Autodesk Inventor part; units mm, degrees
ref_plane "YZ Plane" through (0, 0, 0) normal (1, 0, 0) x (0, 1, 0)
ref_plane "XZ Plane" through (0, 0, 0) normal (0, 1, 0) x (-1, 0, 0)
sketch "Sketch3" plane through (0, 0, 0) normal (0, 0, 1) x (1, 0, 0)
  line L0 (0, -9.525) -> (9.525, -9.525)
  line L1 (9.525, -9.525) -> (9.525, 0)
  line L2 (0, 0) -> (0, -9.525) construction
  line L3 (0, 0) -> (9.525, 0) construction
  line L4 (0, -9.525) -> (-9.525, -9.525)
  line L5 (-9.525, -9.525) -> (-9.525, 0)
  line L6 (9.525, 0) -> (73.025, 0)
  line L7 (-187.325, 0) -> (-187.325, 19.05)
  line L8 (-187.325, 0) -> (-9.525, 0)
  line L9 (73.025, 0) -> (73.025, 19.05)
  line L10 (73.025, 19.05) -> (-187.325, 19.05)
  dimension "d0" = 9.525
  dimension "d1" = 9.525
  dimension "d6" = 63.5
  dimension "d8" = 19.05
  dimension "d9" = 177.8
extrude "Extrusion1" add sketch "Sketch3" along normal mid plane 355.6
sketch "Sketch4" plane through (0, 0, 177.8) normal (0, 0, 1) x (1, 0, 0)
  line L0 (-187.325, 19.05) -> (73.025, 19.05) construction
  line L1 (0, 19.05) -> (0, -9.525) construction
  line L2 (9.525, -9.525) -> (-9.525, -9.525) construction
  line L3 (0, -9.525) -> (-22.225, -9.525)
  line L4 (-22.225, -9.525) -> (-22.225, 19.05)
  line L5 (-22.225, 19.05) -> (0, 19.05)
  line L6 (187.325, 19.05) -> (-73.025, 19.05) construction
  line L7 (0, -9.525) -> (22.225, -9.525)
  line L8 (22.225, -9.525) -> (22.225, 19.05)
  line L9 (0, 19.05) -> (22.225, 19.05)
  point P0 (0, 0)
  dimension "d12" = 22.225
extrude "Extrusion2" add sketch "Sketch4" along normal blind 12.7
mirror "Mirror1" about plane through (0, 0, 0) normal (0, 0, 1) of "Extrusion2"
sketch "Sketch6" plane through (-187.325, 0, -177.8) normal (0, -1, 0) x (1, 0, 0)
  line L0 (82.55, 165.1) -> (88.9, 165.1)
  line L1 (88.9, 165.1) -> (88.9, 190.5)
  line L2 (88.9, 190.5) -> (82.55, 190.5)
  line L3 (82.55, 190.5) -> (82.55, 165.1)
  line L4 (82.55, 165.1) -> (88.9, 190.5) construction
  line L5 (88.9, 165.1) -> (82.55, 190.5) construction
  line L6 (177.8, 0) -> (177.8, 355.6)
  point P0 (187.325, 177.8)
  point P1 (85.725, 177.8)
  dimension "d16" = 12.7
  dimension "d18" = 6.35
  dimension "d19" = 88.9
extrude "Extrusion3" cut sketch "Sketch6" against normal through all
sketch "Sketch7" plane through (0, 0, 177.8) normal (0, 0, 1) x (1, 0, 0)
  line L0 (-187.325, 19.05) -> (-22.225, 19.05)
  line L1 (-161.925, 19.05) -> (-117.475, 19.05)
  line L2 (-117.475, 19.05) -> (-117.475, -3.81)
  line L3 (-117.475, -3.81) -> (-161.925, -3.81)
  line L4 (-161.925, -3.81) -> (-161.925, 19.05)
  line L5 (-187.325, 19.05) -> (-187.325, 0)
  point P0 (0, 0)
  dimension "d22" = 44.45
  dimension "d23" = 22.86
  dimension "d24" = 25.4
extrude "Extrusion4" add sketch "Sketch7" along normal blind 12.7
mirror "Mirror2" about plane through (0, 0, 0) normal (0, 0, 1) of "Extrusion4"
sketch "Sketch9" plane through (73.025, 0, 177.8) normal (1, 0, 0) x (0, 0, -1)
  line L0 (355.6, 19.05) -> (0, 19.05)
  line L1 (50.8, 19.05) -> (63.5, 19.05)
  line L2 (63.5, 19.05) -> (63.5, 12.7)
  line L3 (63.5, 12.7) -> (50.8, 12.7)
  line L4 (50.8, 12.7) -> (50.8, 19.05)
  line L5 (0, 0) -> (0, 19.05)
  point P0 (177.8, 0)
  dimension "d28" = 12.7
  dimension "d29" = 6.35
  dimension "d30" = 50.8
extrude "Extrusion5" cut sketch "Sketch9" against normal through all
mirror "Mirror3" about plane through (0, 0, 0) normal (0, 0, 1) of "Extrusion5"
sketch "Sketch12" plane through (73.025, 0, 177.8) normal (1, 0, 0) x (0, 0, -1)
  line L0 (355.6, 0) -> (0, 0) construction
  line L1 (88.9, 0) -> (88.9, 16.5009) construction
  line L2 (0, 0) -> (0, 19.05)
  line L3 (50.8, 19.05) -> (0, 19.05)
  line L4 (84.1375, 19.05) -> (84.1375, 12.7)
  line L5 (84.1375, 12.7) -> (80.1624, 12.7)
  line L6 (80.1624, 12.7) -> (80.1624, 6.35)
  line L7 (80.1624, 6.35) -> (88.9, 6.35)
  line L8 (93.6625, 19.05) -> (93.6625, 12.7)
  line L9 (93.6625, 12.7) -> (97.6376, 12.7)
  line L10 (97.6376, 12.7) -> (97.6376, 6.35)
  line L11 (97.6376, 6.35) -> (88.9, 6.35)
  line L12 (84.1375, 19.05) -> (93.6625, 19.05)
  point P0 (177.8, 0)
  dimension "d46" = 88.9
  dimension "d47" = 4.7625
  dimension "d48" = 6.35
  dimension "d49" = 6.35
  dimension "d50" = 8.7376
extrude "Extrusion8" cut sketch "Sketch12" against normal through all
mirror "Mirror4" about plane through (0, 0, 0) normal (0, 0, 1) of "Extrusion8"
split "Split2" plane through (0, 0, 0) removes the side toward (0, 0, -1)
ref_plane "Work Plane1" through (-60.325, 0, 177.8) normal (1, 0, 0) x (0, 0, -1)
properties part number "BandSawJigBottomSpiltA" material "LCP Plastic"
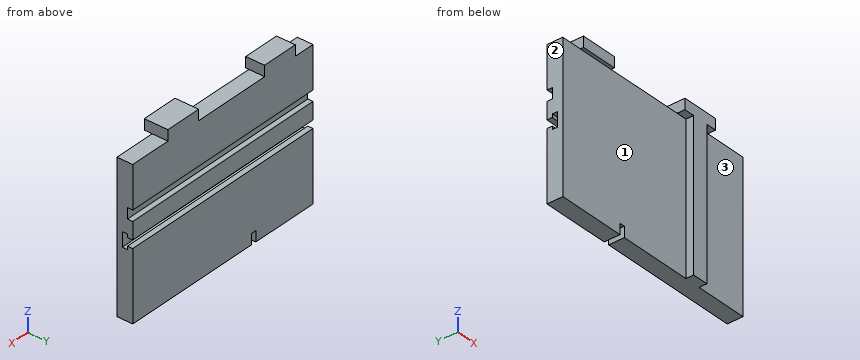
Verification items for the finished model (mm, model axes). Face numbers are marked on the shaded views. A direction names the side the tool comes from. Coordinates: 2 decimals unless noted, no trailing zeros. Order: outer loops, then holes, each group sorted by start corner. A loop starts at its lowest first (then second) coordinate and runs counter-clockwise, first axis right, second up. Notation, with made-up numbers: (80, -17.75) -> (113, -17.75) arc R23 ccw to (113, 8.25) -> close; hole circle Ø4 at (82, 2). An arc over 180 degrees is marked (long way). Use CSV: the item, a comma, the result in double quotes. Start each with the question number.
Q1. Section check D-D, the plane z = 43. Record the cut outline in (x, y) (3 decimals).
Q2. Section check C-C, the plane y = 2.75. Record the cut outline in (x, z) (3 decimals), and give its area (3 significant figures).
Q3. Depth check by flat-ended pin: P1, Ø5, axis at x = 2.5, y = -5, coming from the -Z side; P2, Ø14, axis at x = -146.5, z = 186, coming from the -Y side; P3, Ø6.5, axis at y = 3, z = 187, coming from the -X side (3 decimals); P4, Ø2, axis at x = 23.5, z = 139.5, coming from the -Y side. Enter the tip coordinate at first touch or a pass-through.
Q4. Section check A-A, the plane z = 90.5. Record the cut outline in (x, y) (3 decimals), and give its area (3 significant figures).
Q5. Tool access check on the marked faces 1, 2 and 3. Record the directions out of +Z, -Z, +X, -X, +Y, -Y that give a thin tool (end or side, any length) a straight path to the whole face; none if there is none.
Q6. Thickness scan on line 1 along Z through (x, y) = (0, 16.25); line 2 along Z through (x, y) = (33, 18); line 3 along Z through (x, y) = (5, 11.5). Record the ranges inside material, lowest first.
Q7. Section check B-B, the plane x = -31. Record the cut outline in (y, z).
Returned:
1,outline,"(-187.325, 0) -> (-9.525, 0) -> (-9.525, -9.525) -> (9.525, -9.525) -> (9.525, 0) -> (73.025, 0) -> (73.025, 19.05) -> (-187.325, 19.05) -> close"
2,outline,"(-187.325, 0) -> (-104.775, 0) -> (-104.775, 12.7) -> (-98.425, 12.7) -> (-98.425, 0) -> (73.025, 0) -> (73.025, 177.8) -> (22.225, 177.8) -> (22.225, 190.5) -> (-22.225, 190.5) -> (-22.225, 177.8) -> (-117.475, 177.8) -> (-117.475, 190.5) -> (-161.925, 190.5) -> (-161.925, 177.8) -> (-187.325, 177.8) -> close"
2,area,"47,300 mm^2"
3,P1,"stops at z = 0"
3,P2,"stops at y = -3.81"
3,P3,"stops at x = -161.925"
3,P4,"stops at y = 0"
4,outline,"(-187.325, 0) -> (-9.525, 0) -> (-9.525, -9.525) -> (9.525, -9.525) -> (9.525, 0) -> (73.025, 0) -> (73.025, 6.35) -> (-187.325, 6.35) -> close"
4,area,"1,830 mm^2"
5,face 1,"-Z, -X, -Y"
5,face 2,"+Z, -Z, -X, +Y, -Y"
5,face 3,"-Z, +X, -Y"
6,line 1,"z = 0 to 84.14, 93.66 to 114.3, 127 to 190.5"
6,line 2,"z = 0 to 84.14, 93.66 to 114.3, 127 to 177.8"
6,line 3,"z = 0 to 80.16, 97.64 to 190.5"
7,outline,"(0, 0) -> (19.05, 0) -> (19.05, 84.14) -> (12.7, 84.14) -> (12.7, 80.16) -> (6.35, 80.16) -> (6.35, 97.64) -> (12.7, 97.64) -> (12.7, 93.66) -> (19.05, 93.66) -> (19.05, 114.3) -> (12.7, 114.3) -> (12.7, 127) -> (19.05, 127) -> (19.05, 177.8) -> (0, 177.8) -> close"
